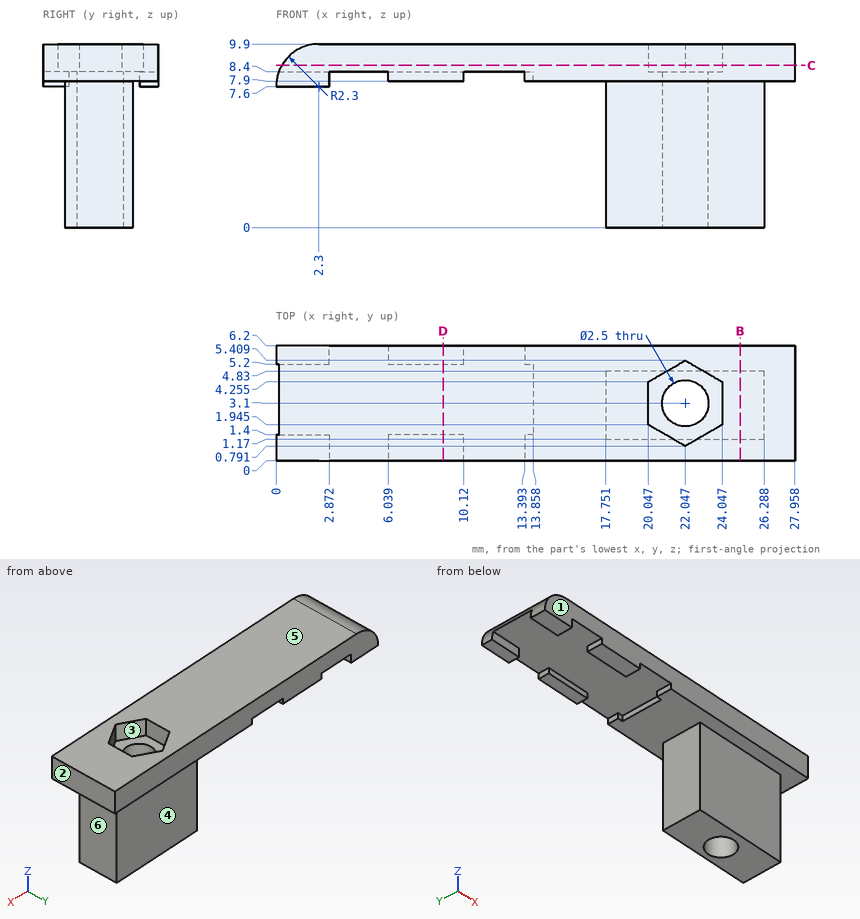
Study the drawing (mm; zero at the part's minimum x, y, z) and answer. A direction names the side the tool comes from. Round coordinates to 2 decimals unless told otherwise and drop trailing zeros. Loops run counter-clockwise (first coordinate to the right, second up) from the corner with the lowest first, then second, coordinate; pieces in that order, holes last. Notation, with made-up numbers: (66.25, 74) - (88.25, 74) arc R15 cw to (88.25, 78) - close; hole circle Ø6 at (22, 11.25). An arc over 180 degrees is marked (long way). Use one line per item in the form item = value. Start each with the question number.
1. The part is cut by section B-B on x = 25. Determine the outline of the cut face in (y, z), then the cut area to 3 significant figures.
2. The part is cut by section C-C on z = 8.75. Determine the outline of the cut face in (x, y) (1 decimal).
3. A tool of negligible diameter and unlimited length cuts with its end or side. For the marked faces 4, 5 and 6, from which of +Z, -Z, +X, -X, +Y, -Y can it reach the whole face along a straight path? Write none if from no direction.
4. For a pull along Y with two mould halves and no side action, classify the marked faces 1, 2 and 3 as pulls with the +Y half, pulls with the -Y half, needs draft (parallel to the pull), parting line crosses it, or undercut.
5. The part is cut by section D-D on x = 9. Determine the outline of the cut face in (y, z).
6. Consider line 1 (X direction, y = 3, z = 5.75); line 2 (Z direction, x = 25, y = 5.75); line 3 (X direction, y = 1, z = 8.5) (1 decimal). Determine where each line is inside the solid, lowest interval first. Write a range as [from, to].
7. Given pin 1 Ø0.9 at (x, z) = (1.5, 8) entering from -Y; pin 2 Ø1.5 at (x, z) = (24, 3.5) entering from +Y; pin 3 Ø3 at (x, y) = (14, 3) entering from -Z; pin 4 Ø2.5 at (x, z) = (21.5, 3.5) entering from -Y, each flat-ended and moving along its own axis, determine where each tip first touches the part or whether it passes through.
Geometry check:
q1.outline = (0, 7.9) - (1.17, 7.9) - (1.17, 0) - (4.83, 0) - (4.83, 7.9) - (6.2, 7.9) - (6.2, 9.9) - (0, 9.9) - close
q1.area = 41.3 mm^2
q2.outline = (0.3, 0) - (28, 0) - (28, 6.2) - (0.3, 6.2) - close; hole (20, 1.9) - (22, 0.8) - (24, 1.9) - (24, 4.3) - (22, 5.4) - (20, 4.3) - close
q3.face_4 = -Z, +X, -X, +Y
q3.face_5 = +Z, +X, -X, +Y, -Y
q3.face_6 = -Z, +X, +Y, -Y
q4.face_1 = pulls with the -Y half
q4.face_2 = needs draft
q4.face_3 = undercut
q5.outline = (0, 7.9) - (1.4, 7.9) - (1.4, 8.4) - (5.2, 8.4) - (5.2, 7.9) - (6.2, 7.9) - (6.2, 9.9) - (0, 9.9) - close
q6.line_1 = [17.75, 20.8], [23.29, 26.29]
q6.line_2 = [7.9, 9.9]
q6.line_3 = [0.2, 21.7], [22.4, 28]
q7.pin_1 = 0
q7.pin_2 = 4.83
q7.pin_3 = 7.9
q7.pin_4 = 1.17
